Autodesk Inventor part; units mm, degrees
ref_plane "BODY_N_XY" through (94, 0, 0) normal (0, 0, -1) x (1, 0, 0)
ref_plane "BODY_N_YZ" through (94, 0, 0) normal (1, 0, 0) x (0, -1, 0)
ref_plane "BODY_N_ZX" through (94, 0, 0) normal (0, -1, 0) x (0, 0, -1)
sketch "Sketch_8" plane through (0, 0, 0) normal (0, 0, 1) x (1, 0, 0)
  line L0 (0, 0) -> (-8, 0)
  line L1 (-8, 0) -> (-8, 3.3865)
  line L2 (-8, 3.3865) -> (-7.3865, 4)
  line L3 (-7.3865, 4) -> (0, 4)
  line L4 (0, 4) -> (0, 0)
  line L5 (0, 0) -> (-8, 0)
revolve "Revolution1" add sketch "Sketch_8" angle 360 about axis through (0, 0, 0) along (1, 0, 0)
thread "Thread1"
sketch "Sketch_9" plane through (0, 0, 0) normal (1, 0, 0) x (0, 0, -1)
  line L0 (-6, 3.6056) -> (-6, -3.6056)
  arc A0 (-6, -3.6056) -> (-3.6056, -6) centre (0, 0) ccw
  line L1 (-3.6056, -6) -> (3.6056, -6)
  arc A1 (3.6056, -6) -> (6, -3.6056) centre (0, 0) ccw
  line L2 (6, -3.6056) -> (6, 3.6056)
  arc A2 (6, 3.6056) -> (3.6056, 6) centre (0, 0) ccw
  line L3 (3.6056, 6) -> (-3.6056, 6)
  arc A3 (-3.6056, 6) -> (-6, 3.6056) centre (0, 0) ccw
extrude "Extrusion1" add sketch "Sketch_9" along normal blind 12.5
sketch "Sketch_6" plane through (12.5, 0, 0) normal (1, 0, 0) x (0, 0, -1)
  circle A0 centre (0, 0) radius 5.5
extrude "Extrusion2" add sketch "Sketch_6" along normal blind 64
sketch "Sketch_10" plane through (76.5, 0, 0) normal (1, 0, 0) x (0, 0, -1)
  line L0 (-6, 3.6056) -> (-6, -3.6056)
  arc A0 (-6, -3.6056) -> (-3.6056, -6) centre (0, 0) ccw
  line L1 (-3.6056, -6) -> (3.6056, -6)
  arc A1 (3.6056, -6) -> (6, -3.6056) centre (0, 0) ccw
  line L2 (6, -3.6056) -> (6, 3.6056)
  arc A2 (6, 3.6056) -> (3.6056, 6) centre (0, 0) ccw
  line L3 (3.6056, 6) -> (-3.6056, 6)
  arc A3 (-3.6056, 6) -> (-6, 3.6056) centre (0, 0) ccw
extrude "Extrusion3" add sketch "Sketch_10" along normal blind 22.5
sketch "Sketch7" plane through (0, 0, 0) normal (0, 0, 1) x (1, 0, 0)
  line L0 (8, 6) -> (8, 1)
  line L1 (8, -0.1934) -> (5.933, 1)
  line L2 (5.933, 1) -> (5.933, 5.567)
  line L3 (5.933, 5.567) -> (5.5, 6)
  line L4 (5.5, 6) -> (8, 6)
  line L5 (8, 6) -> (8, -0.1934)
revolve "Revolution2" cut sketch "Sketch7" angle 360 about axis through (8, 6, 0) along (0, 1, 0)
thread "Thread2"
sketch "Sketch_7" plane through (0, 0, 0) normal (0, 0, 1) x (1, 0, 0)
  line L0 (81, 6) -> (81, 1)
  line L1 (81, -0.1934) -> (78.933, 1)
  line L2 (78.933, 1) -> (78.933, 5.567)
  line L3 (78.933, 5.567) -> (78.5, 6)
  line L4 (78.5, 6) -> (81, 6)
  line L5 (81, 6) -> (81, -0.1934)
revolve "Revolution3" cut sketch "Sketch_7" angle 360 about axis through (81, 6, 0) along (0, 1, 0)
thread "Thread3"
sketch "Sketch_16" plane through (0, 0, 0) normal (0, 0, 1) x (1, 0, 0)
  line L0 (57.5, 0) -> (-8, 0)
  line L1 (-8, 0) -> (-8, 2)
  line L2 (-8, 2) -> (12.5, 2)
  line L3 (12.5, 2) -> (12.5, 5)
  line L4 (12.5, 5) -> (57.5, 5)
  line L5 (57.5, 5) -> (57.5, 0)
  line L6 (57.5, 0) -> (-8, 0)
revolve "Revolution4" cut sketch "Sketch_16" angle 360 about axis through (57.5, 0, 0) along (1, 0, 0)
sketch "Sketch_3" plane through (0, 0, 0) normal (0, 1, 0) x (-1, 0, 0)
  line L0 (-86, 1.6) -> (-99, 1.6)
  line L1 (-99, 1.6) -> (-99, -1.6)
  line L2 (-99, -1.6) -> (-86, -1.6)
  line L3 (-86, -1.6) -> (-86, 1.6)
extrude "Extrusion4" cut sketch "Sketch_3" along normal mid plane 12
sketch "Sketch_13" plane through (0, 0, 0) normal (0, 0, 1) x (1, 0, 0)
  circle A0 centre (94, 0) radius 1.65
extrude "Extrusion5" cut sketch "Sketch_13" along normal mid plane 12
ref_plane "BODY_N_XY" through (94, 0, 0) normal (0, 0, -1) x (1, 0, 0)
ref_plane "BODY_N_YZ" through (94, 0, 0) normal (1, 0, 0) x (0, -1, 0)
ref_plane "BODY_N_ZX" through (94, 0, 0) normal (0, -1, 0) x (0, 0, -1)
ref_plane "BODY_PIN_XY" through (94, 0, 0) normal (-1, 0, 0) x (0, 0, -1)
ref_plane "BODY_PIN_YZ" through (94, 0, 0) normal (0, 0, -1) x (0, -1, 0)
ref_plane "BODY_PIN_ZX" through (94, 0, 0) normal (0, -1, 0) x (-1, 0, 0)
ref_plane "NUT2_XY" through (86, 0, 0) normal (1, 0, 0) x (0, 0, -1)
ref_plane "NUT2_YZ" through (86, 0, 0) normal (0, 0, -1) x (0, 1, 0)
ref_plane "NUT2_ZX" through (86, 0, 0) normal (0, 1, 0) x (1, 0, 0)
ref_plane "SW1_XY" through (17, 0, 0) normal (1, 0, 0) x (0, 0, -1)
ref_plane "SW1_YZ" through (17, 0, 0) normal (0, 0, -1) x (0, 1, 0)
ref_plane "SW1_ZX" through (17, 0, 0) normal (0, 1, 0) x (1, 0, 0)
ref_plane "SW2_XY" through (72, 0, 0) normal (-1, 0, 0) x (0, 0, -1)
ref_plane "SW2_YZ" through (72, 0, 0) normal (0, 0, -1) x (0, -1, 0)
ref_plane "SW2_ZX" through (72, 0, 0) normal (0, -1, 0) x (-1, 0, 0)
ref_plane "SW_R1_XY" through (17, -11, 0) normal (1, 0, 0) x (0, 0, -1)
ref_plane "SW_R1_YZ" through (17, -11, 0) normal (0, 0, -1) x (0, 1, 0)
ref_plane "SW_R1_ZX" through (17, -11, 0) normal (0, 1, 0) x (1, 0, 0)
ref_plane "SW_R2_XY" through (72, -11, 0) normal (-1, 0, 0) x (0, 0, -1)
ref_plane "SW_R2_YZ" through (72, -11, 0) normal (0, 0, -1) x (0, -1, 0)
ref_plane "SW_R2_ZX" through (72, -11, 0) normal (0, -1, 0) x (-1, 0, 0)
ref_plane "body_XY" through (0, 0, 0) normal (-1, 0, 0) x (0, 0, -1)
ref_plane "body_YZ" through (0, 0, 0) normal (0, 0, -1) x (0, -1, 0)
ref_plane "body_ZX" through (0, 0, 0) normal (0, -1, 0) x (-1, 0, 0)
properties part number "CJ2D10-40Z(1_0)_BODY"
For this review, take the finished solid that the model builds, in its own axes (mm). A direction names the side the tool comes from. Give positions to 0.01 mm unless a question says otherwise; leave off trailing zeros. Order: outer loops, then holes, each group sorted by start corner. A loop starts at its lowest first (then second) coordinate and runs counter-clockwise, first axis right, second up. Notation, with made-up numbers: M 35,22.25 L 71,22.25 A25 cw 71,54.25 Z; hole C 14,86 d4. An arc over 180 degrees is marked long. Answer in a Markdown table with one row per item. Add a question column.
(1) For pin 1 (2.5 mm diameter, centred on y = -1, z = 0, fed in from +X); pin 2 (5 mm diameter, centred on x = 57, y = -3, fed in from +Z); pin 3 (2 mm diameter, centred on x = 40, y = 2.5, fed in from -Z), all flat-tipped, find the tip position at first contact; note any pin that passes through.
(2) Consider section A-A on x = 94. State the section outline as (y, z) points, and give its area (3 significant figures).
(3) Mouldability with a two-part tool opening along Y and no side actions: class faces 4 (the face through (35.32, -1.08, -4.88)), 5 (the face through (92.35, 0.07, -3.77)), 6 (the face through (88, 6, -2)), 7 (the face through (86, 0, 0)) as +Y half, -Y half, draft (parallel to the pull), parting line (faces both ways), or undercut.
(4) Wall thickness on probe 1 along X at (y, z) = (0, 3.1); probe 2 along X at (y, z) = (0, 4.7); probe 3 along Y at (x, z) = (94, -2.6): over which ranges is each line inside the solid? List them lowest first. Write a range as [from, to].
(5) Consider section C-C on x = 8. State the section outline as (y, z) points, and give its area (3 significant figures).
(6) For faces 1 (the face through (2, -2, 0)), 2 (the face through (92.6, -1.4, -1.6)), 3 (the face through (87.6, -4.9, -5)), list the 3-axis set-ups (+Z, -Z, +X, -X, +Y, -Y) from which the entire face can be reached by the end or side of a thin tool; tool diameter is ignored.
(7) Consider section B-B on x = 30. State the section outline as (y, z) points.
Evaluation:
| question | item | result |
|---|---|---|
| 1 | pin 1 | stops at x = 86 |
| 1 | pin 2 | stops at z = 5.48 |
| 1 | pin 3 | stops at z = -5.29 |
| 2 | outline | M -6,-3.61 A7 ccw -3.61,-6 L -1.65,-6 L -1.65,-1.6 L -6,-1.6 Z; M -6,1.6 L -1.65,1.6 L -1.65,6 L -3.61,6 A7 ccw -6,3.61 Z; M 1.65,-6 L 3.61,-6 A7 ccw 6,-3.61 L 6,-1.6 L 1.65,-1.6 Z; M 1.65,1.6 L 6,1.6 L 6,3.61 A7 ccw 3.61,6 L 1.65,6 Z |
| 2 | area | 67.0 mm^2 |
| 3 | face 4 | undercut |
| 3 | face 5 | undercut |
| 3 | face 6 | +Y half |
| 3 | face 7 | draft |
| 4 | probe 1 | x = [-8, 12.5], [57.5, 92.35], [95.65, 99] |
| 4 | probe 2 | x = [0, 12.5], [57.5, 92.35], [95.65, 99] |
| 4 | probe 3 | y = [-6, -1.65], [1.65, 6] |
| 5 | outline | M -6,-3.61 A7 ccw -3.61,-6 L 3.61,-6 A7 ccw 6,-3.61 L 6,-2.5 L 5.57,-2.07 L 1,-2.07 L 0.85,-1.81 A2 cw long 0.85,1.81 L 1,2.07 L 5.57,2.07 L 6,2.5 L 6,3.61 A7 ccw 3.61,6 L -3.61,6 A7 ccw -6,3.61 Z |
| 5 | area | 103 mm^2 |
| 6 | face 1 | -X |
| 6 | face 2 | +X, +Y, -Y |
| 6 | face 3 | -Z, +X, -X, -Y |
| 7 | outline | C 0,0 d11; hole C 0,0 d10 |
